Work out the finished part from the listing and answer in its coordinate system (mm). Face numbers are marked on the shaded views. A direction names the side the tool comes from. Coordinates: 2 decimals unless noted, no trailing zeros. Loops run counter-clockwise (first coordinate to the right, second up) from the corner with the lowest first, then second, coordinate; pieces in that order, holes last. Notation, with made-up numbers: (20, 69) -> (60, 69) arc R23 ccw to (60, 106) -> close; hole circle Ø6 at (23.5, 24). An arc over 180 degrees is marked (long way). Use a Markdown table: item, result.
from build123d import *

# Parameters (mm, degrees)
SALIENTE_EXTRUIR1_DEPTH = 10
CORTAR_EXTRUIR1_DEPTH   = 2
SALIENTE_EXTRUIR2_DEPTH = 2
CROQUIS5_W              = 4
CROQUIS5_H              = 3
CORTAR_EXTRUIR2_DEPTH   = 3
CROQUIS6_R              = 1.4
CORTAR_EXTRUIR3_DEPTH   = 5


with BuildPart() as part:
    # Croquis2 → Saliente-Extruir1 (new body)
    with BuildSketch(Plane.XY):
        Polygon((-16, 21), (16, 21), (21, 15), (21, -15), (16, -21), (-16, -21), (-21, -15), (-21, 15), align=None)
    extrude(amount=SALIENTE_EXTRUIR1_DEPTH)

    # Croquis3 → Cortar-Extruir1 (cut)
    with BuildSketch(Plane.XY.offset(10)):
        Polygon((-14, 20), (14, 20), (20, 13.004934109), (20, -13.004934109), (14, -20), (-14, -20), (-20, -13.004934109), (-20, 13.004934109), align=None)
    extrude(amount=-CORTAR_EXTRUIR1_DEPTH, mode=Mode.SUBTRACT)

    # Croquis4 → Saliente-Extruir2 (add)
    with BuildSketch(Plane.XY.offset(10)):
        Polygon((-16, -21), (-14, -20), (-20, -13.004934109), (-21, -15), align=None)
        Polygon((-20, 13.004934109), (-14, 20), (-16, 21), (-21, 15), (-21, 12.992008233), align=None)
        Polygon((16, 21), (21, 15), (20, 13.004934109), (14, 20), align=None)
        Polygon((16, -21), (21, -15), (20, -13.004934109), (14, -20), align=None)
    extrude(amount=SALIENTE_EXTRUIR2_DEPTH)

    # Croquis5 → Cortar-Extruir2 (cut)
    with BuildSketch(Plane.XZ.offset(21)):
        with Locations((0, 5)):
            Rectangle(CROQUIS5_W, CROQUIS5_H)
    extrude(amount=-CORTAR_EXTRUIR2_DEPTH, mode=Mode.SUBTRACT)

    # Croquis6 → Cortar-Extruir3 (cut)
    with BuildSketch(Plane(origin=(0, 0, 0), x_dir=(-1, 0, 0), z_dir=(0, 0, -1))):
        with Locations((15.5, 15.5)):
            Circle(CROQUIS6_R)
        with Locations((-15.5, 15.5)):
            Circle(CROQUIS6_R)
        with Locations((15.5, -15.5)):
            Circle(CROQUIS6_R)
        with Locations((-15.5, -15.5)):
            Circle(CROQUIS6_R)
    extrude(amount=-CORTAR_EXTRUIR3_DEPTH, mode=Mode.SUBTRACT)


solid = part.part
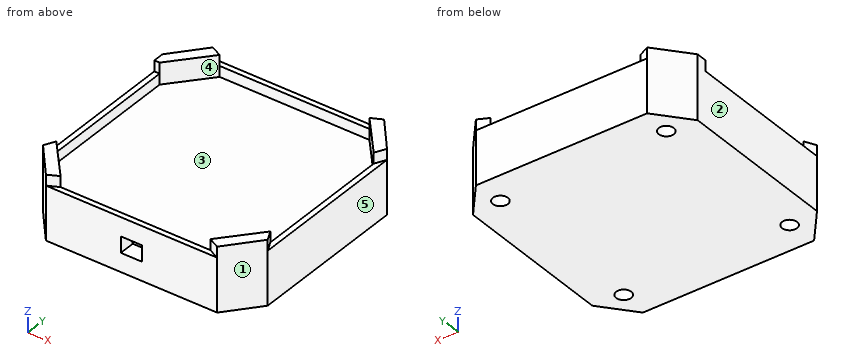
Q1. Section C-C on y = 0.5 is taken. Determine the outline of the cut face in (x, z).
Solved:
| item | result |
|---|---|
| outline | (-21, 0) -> (21, 0) -> (21, 10) -> (20, 10) -> (20, 8) -> (-20, 8) -> (-20, 10) -> (-21, 10) -> close |
Q2. Section B-B on z = 4 is taken. Determine the outline of the cut face in (x, y).
Solved:
| item | result |
|---|---|
| outline | (-21, -15) -> (-16, -21) -> (-2, -21) -> (-2, -18) -> (2, -18) -> (2, -21) -> (16, -21) -> (21, -15) -> (21, 15) -> (16, 21) -> (-16, 21) -> (-21, 15) -> close; hole circle Ø2.8 at (-15.5, -15.5); hole circle Ø2.8 at (-15.5, 15.5); hole circle Ø2.8 at (15.5, -15.5); hole circle Ø2.8 at (15.5, 15.5) |
Q3. Given pin 1 Ø1.4 at (x, y) = (16, 15.5) entering from -Z; pin 2 Ø1.5 at (y, z) = (-20, 5.5) entering from -X; pin 3 Ø0.5 at (x, y) = (20.5, 7) entering from +Z, each flat-ended and moving along its own axis, determine where each tip first touches the part or whether it passes through.
Solved:
| item | result |
|---|---|
| pin 1 | z = 5 |
| pin 2 | x = -17.46 |
| pin 3 | z = 10 |
Q4. Consider line 1 (Y direction, x = -15.5, z = 4); line 2 (Y direction, x = 0, z = 9); line 3 (Y direction, x = -15, z = 0.5). Determine where each line is inside the solid, lowest interval first. Write a range as [from, to].
Solved:
| item | result |
|---|---|
| line 1 | [-21, -16.9], [-14.1, 14.1], [16.9, 21] |
| line 2 | [-21, -20], [20, 21] |
| line 3 | [-21, -16.81], [-14.19, 14.19], [16.81, 21] |
Q5. For the marked faces 4 and 5, determine the directions among +Z, -Z, +X, -X, +Y, -Y from which every point of the face is accessible in a straight line to the end or side of a thin tool.
Solved:
| item | result |
|---|---|
| face 4 | +Z |
| face 5 | +Z, -Z, +X, +Y, -Y |
Q6. Section A-A on z = 9 is taken. Determine the outline of the cut face in (x, y).
Solved:
| item | result |
|---|---|
| outline | (-21, -15) -> (-16, -21) -> (16, -21) -> (21, -15) -> (21, 15) -> (16, 21) -> (-16, 21) -> (-21, 15) -> close; hole (-20, -13) -> (-14, -20) -> (14, -20) -> (20, -13) -> (20, 13) -> (14, 20) -> (-14, 20) -> (-20, 13) -> close |
Q7. Determine the mould class of the marked faces 1, 2 and 3 for opening direction Y: pulls with the +Y half, pulls with the -Y half, needs draft (parallel to the pull), parting line crosses it, or undercut.
Solved:
| item | result |
|---|---|
| face 1 | pulls with the -Y half |
| face 2 | needs draft |
| face 3 | undercut |
